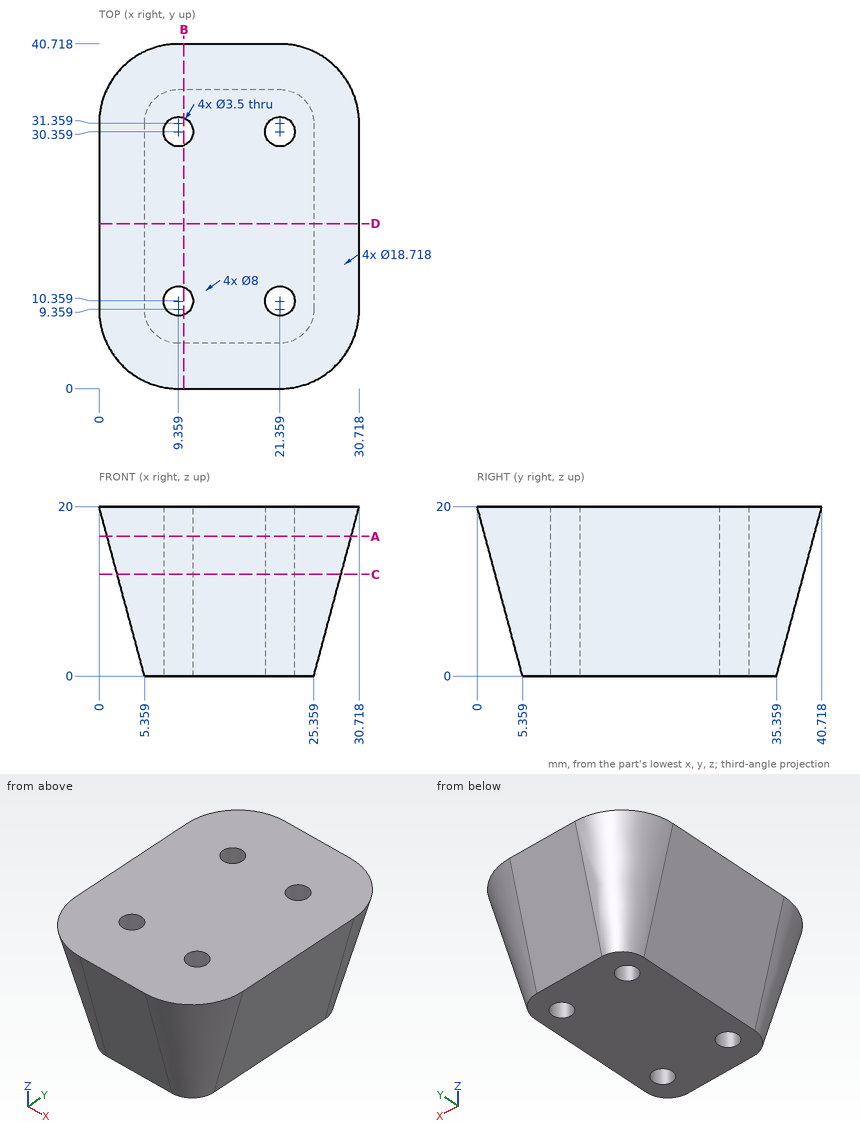
Job drawing, mm, ordinate dimensions from the low corner. One solid piece. Round coordinates to 2 decimals unless told otherwise and drop trailing zeros. Loops run counter-clockwise (first coordinate to the right, second up) from the corner with the lowest first, then second, coordinate; pieces in that order, holes last. Notation, with made-up numbers: (41, 65.5) -> (66, 65.5) arc R16 cw to (66, 71.5) -> close; hole circle Ø5 at (4.25, 49.5). An arc over 180 degrees is marked (long way). Use CSV: the item, a comma, the result in double quotes. Start each with the question number.
Q1. Drill centre lines: L1, parallel to X at y = 9, z = 15.5; L2, parallel to Y at x = 22, z = 5.5 (1 decimal); L3, parallel to X at y = 10, z = 8.75. Where is each one in solid material? Low to high.
Q2. Saw through at C-C on z = 12. Give the cut face in (x, y).
Q3. Saw through at B-B on x = 10. Give the cut face in (y, z).
Q4. Saw through at D-D on y = 19.5. Give the cut face in (x, z), and give its area (3 significant figures).
Q5. Flat gauge pins, fed straight in: pin 1 Ø5 at (y, z) = (10, 15.5) entering from +X; pin 2 Ø10 at (y, z) = (24.5, 13.5) entering from -X; pin 3 Ø1.5 at (y, z) = (20.5, 14.5) entering from +X. Where does each tip first touch, or does it go through?
Q6. Saw through at A-A on z = 16.5. Give the cut face in (x, y), and give its area (3 significant figures).
Solutions:
1,L1,"x = 1.21 to 8.26, 10.46 to 20.26, 22.46 to 29.5"
1,L2,"y = 3.9 to 8.7, 12 to 28.7, 32 to 36.8"
1,L3,"x = 3.01 to 7.65, 11.07 to 19.65, 23.07 to 27.7"
2,outline,"(2.14, 9.36) arc R7.22 ccw to (9.36, 2.14) -> (21.36, 2.14) arc R7.22 ccw to (28.57, 9.36) -> (28.57, 31.36) arc R7.22 ccw to (21.36, 38.57) -> (9.36, 38.57) arc R7.22 ccw to (2.14, 31.36) -> close; hole circle Ø3.5 at (9.36, 10.36); hole circle Ø3.5 at (9.36, 30.36); hole circle Ø3.5 at (21.36, 10.36); hole circle Ø3.5 at (21.36, 30.36)"
3,outline,"(0, 20) -> (5.36, 0) -> (8.73, 0) -> (8.73, 20) -> close; (11.99, 0) -> (28.73, 0) -> (28.73, 20) -> (11.99, 20) -> close; (31.99, 0) -> (35.36, 0) -> (40.72, 20) -> (31.99, 20) -> close"
4,outline,"(0, 20) -> (5.36, 0) -> (25.36, 0) -> (30.72, 20) -> close"
4,area,"507 mm^2"
5,pin 1,"stops at x = 30.18"
5,pin 2,"stops at x = 0.4"
5,pin 3,"stops at x = 29.45"
6,outline,"(0.94, 9.36) arc R8.42 ccw to (9.36, 0.94) -> (21.36, 0.94) arc R8.42 ccw to (29.78, 9.36) -> (29.78, 31.36) arc R8.42 ccw to (21.36, 39.78) -> (9.36, 39.78) arc R8.42 ccw to (0.94, 31.36) -> close; hole circle Ø3.5 at (9.36, 10.36); hole circle Ø3.5 at (9.36, 30.36); hole circle Ø3.5 at (21.36, 10.36); hole circle Ø3.5 at (21.36, 30.36)"
6,area,"1,020 mm^2"
